The model under review builds one solid part; all positions refer to its coordinate system, in mm. A direction names the side the tool comes from. Round coordinates to 2 decimals unless told otherwise and drop trailing zeros. Order: outer loops, then holes, each group sorted by start corner. A loop starts at its lowest first (then second) coordinate and runs counter-clockwise, first axis right, second up. Notation, with made-up numbers: M 85.25,45.25 L 136.25,45.25 A19 cw 136.25,64.25 Z; hole C 71.5,64 d4. An arc over 180 degrees is marked long. Answer as a JSON object with one key per item and string values. Group by question number.
1) To check wall thickness, follow line 1 (Y direction, x = 27.5, z = 13.75); line 2 (X direction, y = 5.5, z = 10); line 3 (Y direction, x = 27.5, z = 5.25). State the ranges of each line that lie inside material, in increasing order.
2) Insertion check: pin 1 Ø7.5 at (x, y) = (-3.5, 1) entering from +Z; pin 2 Ø3.5 at (x, y) = (29, 15) entering from -Z; pin 3 Ø4 at (x, z) = (-8, 5.5) entering from -Y. Each pin has a flat end and moves straight along its axis. Give the tip position at first contact, or say it passes through.
3) Consider section D-D, the plane y = 17. Write out the cut boundary in (x, z).
4) Consider section C-C, the plane z = 15.25. Write out the cut boundary in (x, y).
5) Consider section A-A, the plane x = 27.5. Write out the cut boundary in (y, z), then the cut area to 3 significant figures.
6) The part is to be moulded in two halves that separate along X. For faces 1 (the cylindrical face through (18.93, -23.5, 8.62)), 2 (the flat face through (-5, -9.5, 4)), 3 (the cylindrical face through (-13.169, 0.133, 11.597)), say which applies: +X half, -X half, draft (parallel to the pull), parting line (faces both ways), or undercut.
7) For faces 4 (the flat face through (24, -17, 6.4)), 5 (the cylindrical face through (-11.47, 0.13, 12.62)), 6 (the cylindrical face through (-14.49, 0.13, 2.85)), list the 3-axis set-ups (+Z, -Z, +X, -X, +Y, -Y) from which the entire face can be reached by the end or side of a thin tool; tool diameter is ignored.
```python
from build123d import *

# Parameters (mm, degrees)
BASE_SKETCH_W           = 35
BASE_SKETCH_H           = 19
BASE_DEPTH              = 5
HINGE_SKETCH_W          = 7
HINGE_SKETCH_H          = 19
HINGE_BODY_DEPTH        = 9
HINGE_HOLE_D            = 3.6
DOOR_BODY_SKETCH_W      = 20
DOOR_BODY_SKETCH_H      = 50
DOOR_BODY_DEPTH         = 12
DOOR_SCREWS_D           = 6.6
DOOR_SCREWS_CBORE_D     = 11
DOOR_SCREWS_CBORE_DEPTH = 6.4
HINGE_ROUND_R           = 3.99
HINGE_BODY_ROUND_R      = 10
DOOR_CORNERS_ROUND_R    = 5
DOOR_BODY_LINE_R        = 3


with BuildPart() as part:
    # Base sketch → Base (new body)
    with BuildSketch(Plane.XY):
        Rectangle(BASE_SKETCH_W, BASE_SKETCH_H)
        Polygon((17.5, 25), (17.5, 9.5), (17.5, -9.5), (17.5, -25), (37.5, -25), (37.5, 25), align=None)
    extrude(amount=BASE_DEPTH)

    # Hinge sketch → Hinge body (add)
    with BuildSketch(Plane.XY.offset(5)):
        with Locations((-14, 0)):
            Rectangle(HINGE_SKETCH_W, HINGE_SKETCH_H)
    extrude(amount=HINGE_BODY_DEPTH)

    # Hinge hole (through all)
    with Locations(Plane(origin=(0, -9.5, 0), x_dir=(-1, 0, 0), z_dir=(0, -1, 0))):
        with Locations((14, -10)):
            Hole(HINGE_HOLE_D / 2)

    # Door body sketch → Door body (add)
    with BuildSketch(Plane.XY.offset(5)):
        with Locations((27.5, 0)):
            Rectangle(DOOR_BODY_SKETCH_W, DOOR_BODY_SKETCH_H)
    extrude(amount=DOOR_BODY_DEPTH)

    # Door screws (through all)
    with Locations(Plane(origin=(0, 0, 0), x_dir=(-1, 0, 0), z_dir=(0, 0, -1))):
        with Locations((-27.5, 17), (-27.5, -17)):
            CounterBoreHole(DOOR_SCREWS_D / 2, DOOR_SCREWS_CBORE_D / 2, DOOR_SCREWS_CBORE_DEPTH)

    # Hinge round
    # the kernel refuses this fillet: 3.99 mm, written as the material it takes off along each edge
    with BuildSketch(Plane(origin=(-17.5, -19.475, 14), x_dir=(0, 0, -1), z_dir=(0, 1, 0)), Plane(origin=(-10.5, 19.475, 14), x_dir=(0, 0, -1), z_dir=(0, -1, 0))) as hinge_round_piece_1:
        with BuildLine():
            CenterArc((HINGE_ROUND_R, -HINGE_ROUND_R), HINGE_ROUND_R, 90, 90)
            Line((0, -HINGE_ROUND_R), (0, 0))
            Line((0, 0), (HINGE_ROUND_R, 0))
        make_face()
    extrude(amount=38.95, mode=Mode.SUBTRACT)

    # Hinge body round
    hinge_body_round_edges = [part.edges().sort_by_distance(p)[0] for p in [
        (-17.5, 0, 0),
    ]]
    fillet(hinge_body_round_edges, radius=HINGE_BODY_ROUND_R)

    # Door corners round
    door_corners_round_edges = [part.edges().sort_by_distance(p)[0] for p in [
        (17.5, 25, 8.5),
        (37.5, 25, 8.5),
        (37.5, -25, 8.5),
        (17.5, -25, 8.5),
    ]]
    fillet(door_corners_round_edges, radius=DOOR_CORNERS_ROUND_R)

    # Door body line
    door_body_line_edges = [part.edges().sort_by_distance(p)[0] for p in [
        (17.5, 9.5, 2.5),
        (17.5, -9.5, 2.5),
    ]]
    fillet(door_body_line_edges, radius=DOOR_BODY_LINE_R)


solid = part.part
```
Results list:
{
 "1": {"line 1": "-25 to -20.3, -13.7 to 13.7, 20.3 to 25", "line 2": "-17.5 to -15.8, -12.2 to -10.5, 17.5 to 37.5", "line 3": "-25 to -22.5, -11.5 to 11.5, 22.5 to 25"},
 "2": {"pin 1": "z = 5", "pin 2": "z = 6.4", "pin 3": "y = -9.5"},
 "3": {"outline": "M 17.5,0 L 22,0 L 22,6.4 L 24.2,6.4 L 24.2,17 L 17.5,17 Z; M 30.8,6.4 L 33,6.4 L 33,0 L 37.5,0 L 37.5,17 L 30.8,17 Z"},
 "4": {"outline": "M 17.5,-20 A5 ccw 22.5,-25 L 32.5,-25 A5 ccw 37.5,-20 L 37.5,20 A5 ccw 32.5,25 L 22.5,25 A5 ccw 17.5,20 Z; hole C 27.5,-17 d6.6; hole C 27.5,17 d6.6"},
 "5": {"outline": "M -25,0 L -22.5,0 L -22.5,6.4 L -20.3,6.4 L -20.3,17 L -25,17 Z; M -13.7,6.4 L -11.5,6.4 L -11.5,0 L 11.5,0 L 11.5,6.4 L 13.7,6.4 L 13.7,17 L -13.7,17 Z; M 20.3,6.4 L 22.5,6.4 L 22.5,0 L 25,0 L 25,17 L 20.3,17 Z", "area": "569 mm^2"},
 "6": {"face 1": "-X half", "face 2": "draft", "face 3": "undercut"},
 "7": {"face 4": "-Z", "face 5": "+Z, +Y, -Y", "face 6": "-Z, -X, +Y, -Y"}
}
